from build123d import *

# Parameters (mm, degrees)
SKETCH_2_W          = 24
SKETCH_2_H          = 5
SKETCH_2_R          = 1.7
EXTRUDE_1_DEPTH     = 3
FILLET_2_R          = 6.8
EXTRUDE_START       = 2
SKETCH_4_W          = 8.7
SKETCH_4_H          = 40
SKETCH_4_R          = 1.7
SKETCH_4_H_2        = 12
EXTRUDE_2_DEPTH     = 2
FILLET_3_R          = 3.4
SKETCH_5_R          = 1.9
SKETCH_5_R_2        = 1.8
CUT_EXTRUDE_1_DEPTH = 10


with BuildPart() as part:
    # 草图2 → 凸台-拉伸1 (new body)
    # profile 1 of 7: a face of its own
    with BuildSketch(Plane(origin=(0, 0, 0), x_dir=(1, 0, 0), z_dir=(0, 1, 0))):
        with BuildLine():
            Line((25, -8), (12, -8))
            Line((12, -8), (12, -15))
            Line((12, -15), (23.3, -15))
            ThreePointArc((23.3, -15), (23.797918472, -13.797918472), (25, -13.3))
            Line((25, -13.3), (25, -8))
        make_face()
    # profile 2 of 7: a face of its own
    with BuildSketch(Plane(origin=(0, 0, 0), x_dir=(1, 0, 0), z_dir=(0, 1, 0))):
        with BuildLine():
            Line((23.3, -15), (12, -15))
            Line((12, -15), (12, -20))
            Line((12, -20), (30, -20))
            Line((30, -20), (30, -8))
            Line((30, -8), (25, -8))
            Line((25, -8), (25, -13.3))
            ThreePointArc((25, -13.3), (26.202081528, -13.797918472), (26.7, -15))
            ThreePointArc((26.7, -15), (25, -16.7), (23.3, -15))
        make_face()
    # profile 3 of 7: a face of its own
    with BuildSketch(Plane(origin=(0, 0, 0), x_dir=(1, 0, 0), z_dir=(0, 1, 0))):
        with Locations((0, -17.5)):
            Rectangle(SKETCH_2_W, SKETCH_2_H)
    # profile 4 of 7: a face of its own
    with BuildSketch(Plane(origin=(0, 0, 0), x_dir=(1, 0, 0), z_dir=(0, 1, 0))):
        Polygon((12, 15), (-12, 15), (-12, -15), (12, -15), (12, -8), align=None)
        with Locations(Location((-7.425, -7.425, 0), (0, 0, 270))):
            Circle(SKETCH_2_R, mode=Mode.SUBTRACT)
        with Locations(Location((7.425, -7.425, 0), (0, 0, 270))):
            Circle(SKETCH_2_R, mode=Mode.SUBTRACT)
        with Locations(Location((-7.425, 7.425, 0), (0, 0, 270))):
            Circle(SKETCH_2_R, mode=Mode.SUBTRACT)
        with Locations(Location((7.425, 7.425, 0), (0, 0, 270))):
            Circle(SKETCH_2_R, mode=Mode.SUBTRACT)
    # profile 5 of 7: a face of its own
    with BuildSketch(Plane(origin=(0, 0, 0), x_dir=(1, 0, 0), z_dir=(0, 1, 0))):
        with Locations((0, 17.5)):
            Rectangle(SKETCH_2_W, SKETCH_2_H)
    # profile 6 of 7: a face of its own
    with BuildSketch(Plane(origin=(0, 0, 0), x_dir=(1, 0, 0), z_dir=(0, 1, 0))):
        with BuildLine():
            Line((-12, 15), (-23.3, 15))
            ThreePointArc((-23.3, 15), (-23.797918472, 13.797918472), (-25, 13.3))
            Line((-25, 13.3), (-25, -13.3))
            ThreePointArc((-25, -13.3), (-23.797918472, -13.797918472), (-23.3, -15))
            Line((-23.3, -15), (-12, -15))
            Line((-12, -15), (-12, 15))
        make_face()
    # profile 7 of 7: a face of its own
    with BuildSketch(Plane(origin=(0, 0, 0), x_dir=(1, 0, 0), z_dir=(0, 1, 0))):
        with BuildLine():
            ThreePointArc((-25, 13.3), (-26.202081528, 16.202081528), (-23.3, 15))
            Line((-23.3, 15), (-12, 15))
            Line((-12, 15), (-12, 20))
            Line((-12, 20), (-30, 20))
            Line((-30, 20), (-30, -20))
            Line((-30, -20), (-12, -20))
            Line((-12, -20), (-12, -15))
            Line((-12, -15), (-23.3, -15))
            ThreePointArc((-23.3, -15), (-26.202081528, -16.202081528), (-25, -13.3))
            Line((-25, -13.3), (-25, 13.3))
        make_face()
    extrude(amount=EXTRUDE_1_DEPTH)

    # 圆角2
    fillet_2_edges = [part.edges().sort_by_distance(p)[0] for p in [
        (12, 1.5, 8),
    ]]
    fillet(fillet_2_edges, radius=FILLET_2_R)

    # 草图4 → 凸台-拉伸2 (add)
    # profile 1 of 2: a face of its own
    with BuildSketch(Plane.XZ.offset(EXTRUDE_START)):
        with Locations((-25.65, 0)):
            Rectangle(SKETCH_4_W, SKETCH_4_H)
        with Locations(Location((-25, 15, 0), (0, 0, 270))):
            Circle(SKETCH_4_R, mode=Mode.SUBTRACT)
        with Locations(Location((-25, -15, 0), (0, 0, 270))):
            Circle(SKETCH_4_R, mode=Mode.SUBTRACT)
    # profile 2 of 2: a face of its own
    with BuildSketch(Plane.XZ.offset(EXTRUDE_START)):
        with Locations((25.65, 14)):
            Rectangle(SKETCH_4_W, SKETCH_4_H_2)
        with Locations(Location((25, 15, 0), (0, 0, 270))):
            Circle(SKETCH_4_R, mode=Mode.SUBTRACT)
    extrude(amount=-EXTRUDE_2_DEPTH)

    # 圆角3
    fillet_3_edges = [part.edges().sort_by_distance(p)[0] for p in [
        (12, 1.5, -20),
        (30, 0.5, 8),
        (30, 0.5, 20),
        (-30, 0.5, 20),
        (-30, 0.5, -20),
    ]]
    fillet(fillet_3_edges, radius=FILLET_3_R)

    # 草图5 → 切除-拉伸1 (cut)
    with BuildSketch(Plane(origin=(0, 3, 0), x_dir=(1, 0, 0), z_dir=(0, 1, 0))):
        with Locations(Location((-7.425, -7.425, 0), (0, 0, 270))):
            Circle(SKETCH_5_R)
        with Locations(Location((-7.425, 7.425, 0), (0, 0, 270))):
            Circle(SKETCH_5_R_2)
    extrude(amount=-CUT_EXTRUDE_1_DEPTH, mode=Mode.SUBTRACT)


solid = part.part
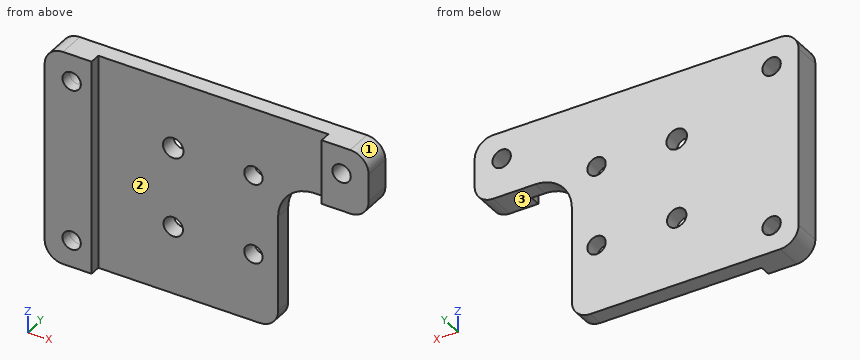
Input: part model. Units: mm. Frame: model coordinates. Face numbers are marked on the shaded views. A direction names the side the tool comes from. Round coordinates to 2 decimals unless told otherwise and drop trailing zeros. Order: outer loops, then holes, each group sorted by start corner. A loop starts at its lowest first (then second) coordinate and runs counter-clockwise, first axis right, second up. Notation, with made-up numbers: (-31, -22) - (6, -22) arc R29 ccw to (6, 8) - close; hole circle Ø9 at (-10.5, 43.5). An arc over 180 degrees is marked (long way). Use a Markdown table: item, result.
1. Material intervals for probe 1 along Z at (x, y) = (-25, 2.3); probe 2 along X at (y, z) = (0.65, 15); probe 3 along X at (y, z) = (-1, 15), sorted ascending.
Evaluation:
| item | result |
|---|---|
| probe 1 | -20 to -16.7, -13.3 to 13.3, 16.7 to 20 |
| probe 2 | -30 to -26.7, -23.3 to 23.3, 26.7 to 30 |
| probe 3 | -30 to -26.7, -23.3 to -21.3, 21.3 to 23.3, 26.7 to 30 |
2. Section A-A on y = -1. Return the cut outline in (x, z).
Evaluation:
| item | result |
|---|---|
| outline | (-30, -16.6) arc R3.4 ccw to (-26.6, -20) - (-21.3, -20) - (-21.3, 20) - (-26.6, 20) arc R3.4 ccw to (-30, 16.6) - close; (21.3, 8) - (26.6, 8) arc R3.4 ccw to (30, 11.4) - (30, 16.6) arc R3.4 ccw to (26.6, 20) - (21.3, 20) - close; hole circle Ø3.4 at (-25, -15); hole circle Ø3.4 at (-25, 15); hole circle Ø3.4 at (25, 15) |
3. First-contact query: pin 1 (4.5 mm diameter, centred on x = -7.425, z = -7.425, fed in from -Y); pin 2 (2.5 mm diameter, centred on x = 7.425, z = 7.425, fed in from -Y); pin 3 (0.9 mm diameter, centred on y = 2, z = -5.5, fed in from +X); pin 4 (1.5 mm diameter, centred on x = 22.5, y = 1, fed in from -Z). Flat tips, straight axial feed; report the tip coordinate or a pass-through.
Evaluation:
| item | result |
|---|---|
| pin 1 | y = 0 |
| pin 2 | through |
| pin 3 | x = 12 |
| pin 4 | z = 8 |
4. Access query for the marked faces 1, 2 and 3. Directions: +Z, -Z, +X, -X, +Y, -Y. A direction counts if a zero-diameter tool reaches every point of the face in a straight line with its end or side. Return the directions, or none.
Evaluation:
| item | result |
|---|---|
| face 1 | +Z, +X, +Y, -Y |
| face 2 | +Z, -Z, -Y |
| face 3 | -Z, +X, +Y, -Y |
5. Section D-D on z = -2. Return the cut outline in (x, y).
Evaluation:
| item | result |
|---|---|
| outline | (-30, -2) - (-21.3, -2) - (-21.3, 0) - (12, 0) - (12, 3) - (-30, 3) - close |
6. Section C-C on x = -1. Return the cut outline in (y, z).
Evaluation:
| item | result |
|---|---|
| outline | (0, -20) - (3, -20) - (3, 20) - (0, 20) - close |
7. Section B-B on y = 2.15. Return the cut outline in (x, z) (3 decimals).
Evaluation:
| item | result |
|---|---|
| outline | (-30, -16.6) arc R3.4 ccw to (-26.6, -20) - (8.6, -20) arc R3.4 ccw to (12, -16.6) - (12, 1.2) arc R6.8 cw to (18.8, 8) - (26.6, 8) arc R3.4 ccw to (30, 11.4) - (30, 16.6) arc R3.4 ccw to (26.6, 20) - (-26.6, 20) arc R3.4 ccw to (-30, 16.6) - close; hole circle Ø3.4 at (-25, -15); hole circle Ø3.4 at (-25, 15); hole circle Ø3.8 at (-7.425, 7.425); hole circle Ø3.6 at (-7.425, -7.425); hole circle Ø3.4 at (7.425, -7.425); hole circle Ø3.4 at (7.425, 7.425); hole circle Ø3.4 at (25, 15) |
